from build123d import *

# Parameters (mm, degrees)
F3_DEPTH      = 19.0510001
F3_DEPTH_BACK = 19.0510001


with BuildPart() as f1:
    # F0 (on Front) → F1 (revolve)
    with BuildSketch(Plane.XZ):
        with BuildLine():
            Line((-38.1, 12.7), (-88.9, 12.7))
            Line((-88.9, 12.7), (-88.9, 0))
            Line((-88.9, 0), (76.2, 0))
            Line((76.2, 0), (76.2, 19.05))
            Line((76.2, 19.05), (0, 19.05))
            ThreePointArc((0, 19.05), (-9.6563855168, 18.2508131011), (-19.05, 15.875))
            ThreePointArc((-19.05, 15.875), (-28.4436144832, 13.4991868989), (-38.1, 12.7))
        make_face()
    revolve(axis=Axis((-6.35, 0, 0), (1, 0, 0)))

    # F2 (on Front) → F3 (cut, two sides)
    with BuildSketch(Plane.XZ) as f3_sk:
        with BuildLine():
            Line((76.2, -1.5875), (76.2, 1.5875))
            Line((76.2, 1.5875), (0, 1.5875))
            ThreePointArc((0, 1.5875), (-1.5875, 0), (0, -1.5875))
            Line((0, -1.5875), (76.2, -1.5875))
        make_face()
    extrude(amount=-F3_DEPTH, mode=Mode.SUBTRACT)
    extrude(f3_sk.sketch, amount=F3_DEPTH_BACK, mode=Mode.SUBTRACT)


solid = f1.part
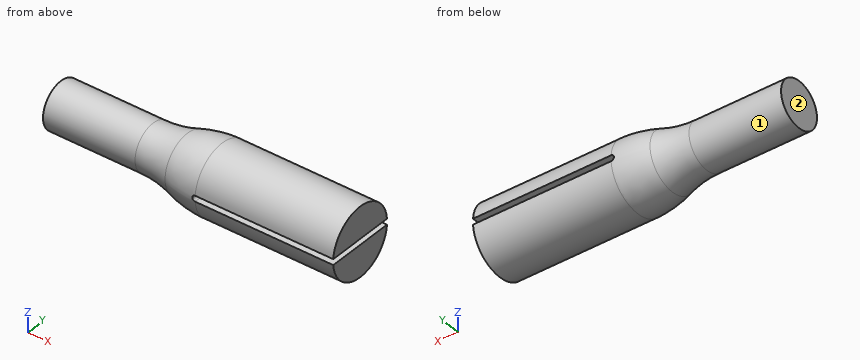
Can you work these out from the model? Positions are in its coordinate system, mm. Face numbers are marked on the shaded views. A direction names the side the tool comes from. Round coordinates to 2 decimals unless told otherwise and drop trailing zeros. Write each loop counter-clockwise with the first axis right and the second up, starting at its lowest first coordinate (ties: lowest second). Pieces come first, ordered by that corner, then holes. Notation, with made-up numbers: (-11, -38) -> (-2, -38) arc R13 cw to (-2, -27) -> close; hole circle Ø4 at (6, 33). An arc over 180 degrees is marked (long way). Use one line per item in the form item = value. Start each with the question number.
Q1. If I drill on probe 1 along Z at (x, y) = (4.5, -10.5); probe 2 along Z at (x, y) = (53.5, 0); probe 3 along Y at (x, z) = (-62.5, -5), over which ranges is the centre line in solid material (lowest first)? Write a range as [from, to].
Q2. Imagine slicing it at A-A (x = 27). Please give me the cut outline in (y, z), then the cut area to 3 significant figures.
Q3. I'm going to push flat-ended pins straight in: P1, Ø4, axis at x = 29, z = 14.5, coming from the -Y side; P2, Ø6, axis at x = -39, y = -14.5, coming from the -Z side; P3, Ø5, axis at x = 2.5, z = 10, coming from the +Y side. Where does each tip first touch, or does it pass through?
Q4. Which directions (+Z, -Z, +X, -X, +Y, -Y) give clear straight access to the entire face, cutting with the end or side of a thin tool? Please do the marked faces 1 and 2.
Q5. Imagine slicing it at C-C (x = -27.5). Please give me the cut outline in (y, z), then the cut area to 3 significant figures.
Q6. Imagine slicing it at B-B (x = -71.5). Please give me the cut outline in (y, z).
Worked out:
q1.probe_1 = [-15.9, -1.59], [1.59, 15.9]
q1.probe_2 = [-19.05, -1.59], [1.59, 19.05]
q1.probe_3 = [-11.67, 11.67]
q2.outline = (-18.98, -1.59) arc R19.05 ccw to (18.98, -1.59) -> close; (-18.98, 1.59) -> (18.98, 1.59) arc R19.05 ccw to start
q2.area = 1,020 mm^2
q3.P1 = -14.38
q3.P2 = -5.39
q3.P3 = 17.51
q4.face_1 = -X
q4.face_2 = +Z, -Z, -X, +Y, -Y
q5.outline = circle Ø27.33 at (0, 0)
q5.area = 587 mm^2
q6.outline = circle Ø25.4 at (0, 0)
